```python
from build123d import *

# Parameters (mm, degrees)
F_3_8_CLEARANCE_HOLE1_D = 10.0838
SKETCH2_R               = 12.7
RF_CONNECTOR_DEPTH      = 25.4


with BuildPart() as part:
    # Sketch1 → Revolve1 (revolve)
    with BuildSketch(Plane.XY, mode=Mode.PRIVATE) as revolve1_sk:
        Polygon((0, 152.4), (19.05, 152.4), (37.34122006, 3.175), (74.083333333, 3.175), (98.425, 76.2), (101.6, 76.2), (76.2, 0), (0, 0), align=None)
    revolve(revolve1_sk.sketch.rotate(Axis((0, 0, 0), (0, 1, 0)), 90), axis=Axis((0, 0, 0), (0, 1, 0)))

    # 3/8 Clearance Hole1 (through all)
    with Locations(Plane(origin=(0, 0, 0), x_dir=(-1, 0, 0), z_dir=(0, -1, 0))):
        with Locations((38.1, -23.493790612), (-38.1, -23.493790612)):
            Hole(F_3_8_CLEARANCE_HOLE1_D / 2)

    # Sketch2 → RF Connector (add)
    with BuildSketch(Plane.XZ):
        with Locations(Location((0, 0, 0), (0, 0, 270))):
            Circle(SKETCH2_R)
    extrude(amount=RF_CONNECTOR_DEPTH)


solid = part.part
```
Geometry: final body of the model. Coordinates: model frame, mm. A direction names the side the tool comes from. Give positions to 0.01 mm unless a question says otherwise; leave off trailing zeros. Loops run counter-clockwise (first coordinate to the right, second up) from the corner with the lowest first, then second, coordinate; pieces in that order, holes last. Notation, with made-up numbers: (-24, -29) -> (-5, -29) arc R20 cw to (-5, -1) -> close; hole circle Ø9 at (58, -30). An arc over 180 degrees is marked (long way). Return JSON: item names as keys, results as strings.
Item 1: Access query for faces 1 (the cylindrical face through (-7.7, -12.5, 10.1)), 2 (the conical face through (76.45, 15.86, 16.98)). Directions: +Z, -Z, +X, -X, +Y, -Y. A direction counts if a zero-diameter tool reaches every point of the face in a straight line with its end or side. Return the directions, or none.
Filled in:
{"face 1": "-Y", "face 2": "+Y"}
Item 2: Section D-D, the plane y = -12. Output: boundary loops of the cut face in (x, z).
Filled in:
{"outline": "circle Ø25.4 at (0, 0)"}
Item 3: Section B-B, the plane z = 0. Output: boundary loops of the cut face in (x, y) (3 decimals).
Filled in:
{"outline": "(-101.6, 76.2) -> (-76.2, 0) -> (-12.7, 0) -> (-12.7, -25.4) -> (12.7, -25.4) -> (12.7, 0) -> (76.2, 0) -> (101.6, 76.2) -> (98.425, 76.2) -> (74.083, 3.175) -> (37.341, 3.175) -> (19.05, 152.4) -> (-19.05, 152.4) -> (-37.341, 3.175) -> (-74.083, 3.175) -> (-98.425, 76.2) -> close"}
Item 4: Pin query (flat end, axial travel): P1, Ø3, axis at x = 54, z = 18, coming from the +Y side (3 decimals); P2, Ø3, axis at x = 51, z = 21, coming from the -Y side; P3, Ø4, axis at x = -66.5, y = 63, coming from the +Z side; P4, Ø1, axis at y = 114.5, z = -24.5, coming from the +X side. Return the tip coordinate at first contact, or that it passes through.
Filled in:
{"P1": "y = 3.175", "P2": "y = 0", "P3": "z = 72.93", "P4": "through"}
Item 5: Mould query, pull axis X, two halves, no side actions, for faces 3 (the cylindrical face through (-35.39, 1.61, 19.24)), 4 (the flat face through (0, 152.4, 0)), 5 (the conical face through (-24.11, 12.17, -76.55)), 6 (the flat face through (-18, 3.175, -34)). Classes: released by +X, released by -X, zero draft, split by the parting line, or undercut.
Filled in:
{"face 3": "undercut", "face 4": "zero draft", "face 5": "split by the parting line", "face 6": "undercut"}
Item 6: Section C-C, the plane y = 26. Output: boundary loops of the cut face in (x, z), plus the area to 3 significant figures.
Filled in:
{"outline": "circle Ø169.73 at (0, 0); circle Ø69.09 at (0, 0); hole circle Ø163.38 at (0, 0)", "area": "5,410 mm^2"}
Item 7: Section A-A, the plane x = 0. Output: boundary loops of the cut face in (y, z) (3 decimals).
Filled in:
{"outline": "(-25.4, -12.7) -> (0, -12.7) -> (0, -76.2) -> (76.2, -101.6) -> (76.2, -98.425) -> (3.175, -74.083) -> (3.175, -37.341) -> (152.4, -19.05) -> (152.4, 19.05) -> (3.175, 37.341) -> (3.175, 74.083) -> (76.2, 98.425) -> (76.2, 101.6) -> (0, 76.2) -> (0, 12.7) -> (-25.4, 12.7) -> close"}
Item 8: Line query: line 1 (X direction, y = 38, z = 1); line 2 (Z direction, x = -18, y = 5); line 3 (Z direction, x = -38.1, y = 1.3). Output: solid intervals per line, ascending.
Filled in:
{"line 1": "-88.86 to -85.69, -33.06 to 33.06, 85.69 to 88.86", "line 2": "-75.76 to -72.49, -32.46 to 32.46, 72.49 to 75.76", "line 3": "-66.49 to 18.45, 28.54 to 66.49"}
